Model file for the job. Use its own axes, mm. Coordinates: 2 decimals unless noted, no trailing zeros. Loops run counter-clockwise (first coordinate to the right, second up) from the corner with the lowest first, then second, coordinate; pieces in that order, holes last.
from build123d import *

# Parameters (mm, degrees)
BOSS_EXTRUDE1_DEPTH      = 4
BOSS_EXTRUDE1_DEPTH_BACK = 4
SKETCH2_R                = 20
SKETCH2_R_2              = 10


with BuildPart() as part:
    # Sketch2 → Boss-Extrude1 (new, two sides: drawn at the far end of the back side and taken through both)
    # profile 1 of 3: a face of its own
    with BuildSketch(Plane(origin=(0, 0, 0), x_dir=(0, 0, -1), z_dir=(1, 0, 0)).offset(-BOSS_EXTRUDE1_DEPTH_BACK)):
        with BuildLine():
            ThreePointArc((20, 0), (0, -20), (-20, 0))
            Line((-20, 0), (-20, -200))
            ThreePointArc((-20, -200), (0, -180), (20, -200))
            Line((20, -200), (20, 0))
        make_face()
    # profile 2 of 3: a face of its own
    with BuildSketch(Plane(origin=(0, 0, 0), x_dir=(0, 0, -1), z_dir=(1, 0, 0)).offset(-BOSS_EXTRUDE1_DEPTH_BACK)):
        Circle(SKETCH2_R)
        Circle(SKETCH2_R_2, mode=Mode.SUBTRACT)
    # profile 3 of 3: a face of its own
    with BuildSketch(Plane(origin=(0, 0, 0), x_dir=(0, 0, -1), z_dir=(1, 0, 0)).offset(-BOSS_EXTRUDE1_DEPTH_BACK)):
        with Locations((0, -200)):
            Circle(SKETCH2_R)
    extrude(amount=BOSS_EXTRUDE1_DEPTH + BOSS_EXTRUDE1_DEPTH_BACK)


solid = part.part
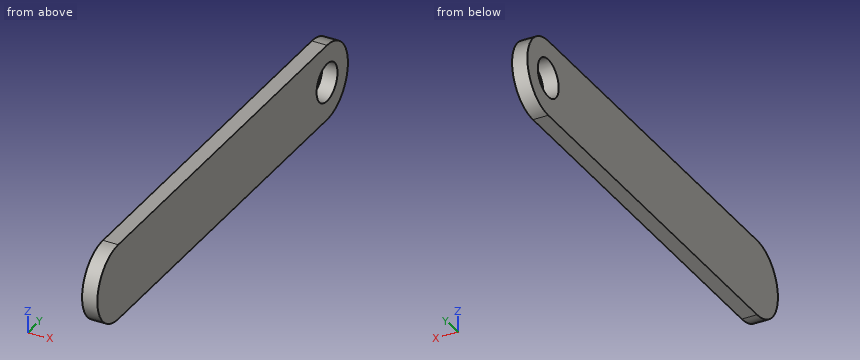
Q1. Slice it at B-B (x = 2). List the corners of the cut face in (y, z), and give its area (3 significant figures).
Answers:
outline: (-200, -20) - (0, -20) arc R20 ccw to (0, 20) - (-200, 20) arc R20 ccw to start; hole circle Ø20 at (0, 0)
area: 8,940 mm2
Q2. Slice it at C-C (y = -4.5). List the corners of the cut face in (x, z), and give its area (3 significant figures).
Answers:
outline: (-4, -20) - (4, -20) - (4, -8.93) - (-4, -8.93) - close; (-4, 8.93) - (4, 8.93) - (4, 20) - (-4, 20) - close
area: 177 mm2
Q3. Drill centre lines: line 1 (Y direction, x = -0.25, z = 0); line 2 (Y direction, x = 3.25, z = 8); line 3 (Y direction, x = -3.25, z = -14.5). Where is each one in solid material? Low to high.
Answers:
line 1: y = -220 to -10, 10 to 20
line 2: y = -218.33 to -6, 6 to 18.33
line 3: y = -213.77 to 13.77
Q4. Slice it at D-D (z = -15). List the corners of the cut face in (x, y).
Answers:
outline: (-4, -213.23) - (4, -213.23) - (4, 13.23) - (-4, 13.23) - close
Q5. Flat gauge pins, fed straight in: P1, Ø1, axis at x = -1.5, z = 5.5, coming from the +Y side; P2, Ø1, axis at x = -1.5, z = -9, coming from the +Y side. Where does each tip first touch, or does it go through?
Answers:
P1: stops at y = 19.36
P2: stops at y = 18.1
Q6. Slice it at A-A (z = 0). List the corners of the cut face in (x, y).
Answers:
outline: (-4, -220) - (4, -220) - (4, -10) - (-4, -10) - close; (-4, 10) - (4, 10) - (4, 20) - (-4, 20) - close
